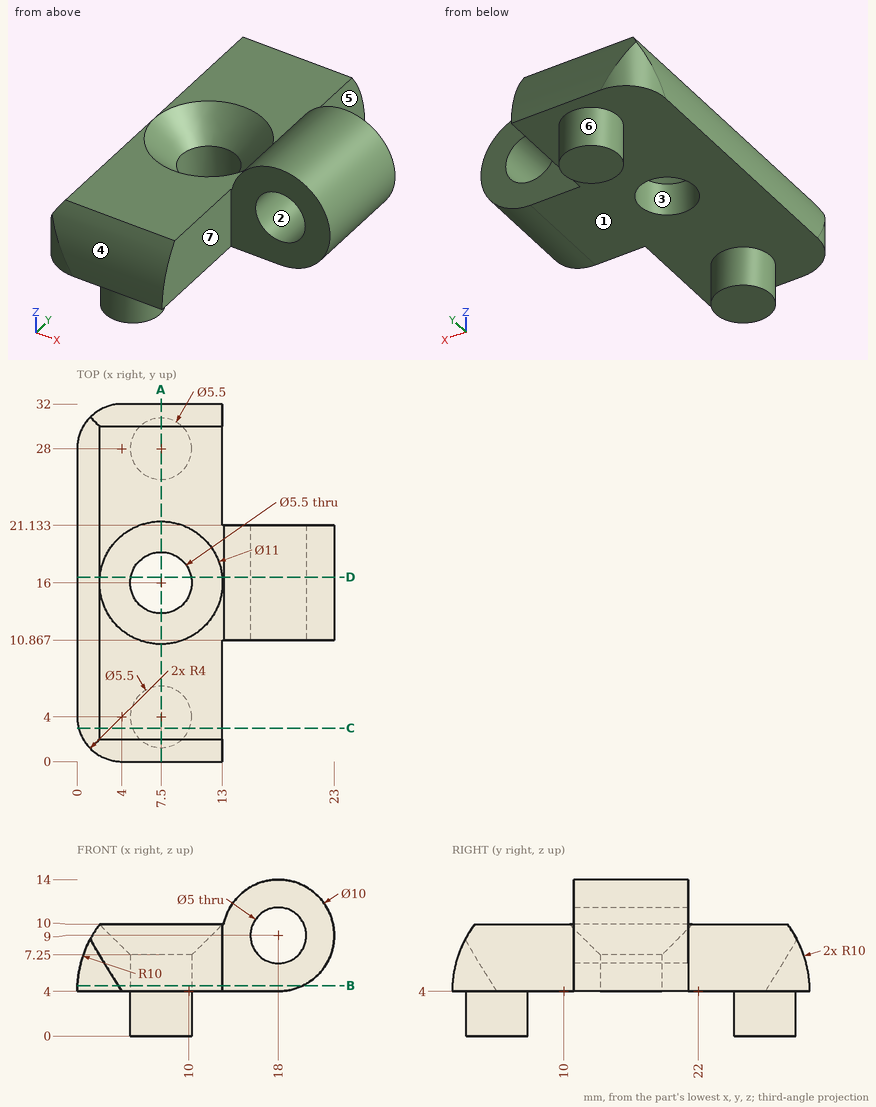
The figure shows three views and two pictorial views of one solid part (mm, origin at its lowest corner). Answer the questions. A direction names the side the tool comes from. Give positions to 0.01 mm unless a question says otherwise; leave off trailing zeros. Loops run counter-clockwise (first coordinate to the right, second up) from the corner with the lowest first, then second, coordinate; pieces in that order, holes last. Notation, with made-up numbers: (81.25, -28.75) - (133.25, -28.75) arc R21 ccw to (133.25, -10.75) - close; hole circle Ø6 at (4, 0.25). An arc over 180 degrees is marked (long way). Use one line per item in the form item = value.
1. Section D-D on y = 16.5 is taken. Count the separate pieces of the cut face and the enclosed holes in it.
Calculated:
separate_pieces = 2
enclosed_holes = 1
2. Section B-B on z = 4.5 is taken. Give the vertices of the cut face in (x, y).
Calculated:
outline = (0.01, 3.68) arc R4 ccw to (3.68, 0.01) - (13, 0.01) - (13, 10.87) - (20.18, 10.87) - (20.18, 21.13) - (13, 21.13) - (13, 31.99) - (3.68, 31.99) arc R4 ccw to (0.01, 28.32) - close; hole circle Ø5.5 at (7.5, 16)
3. Section C-C on y = 3 is taken. Give the vertices of the cut face in (x, z).
Calculated:
outline = (0.13, 4) - (4.94, 4) - (4.94, 0) - (10.06, 0) - (10.06, 4) - (13, 4) - (13, 10) - (2, 10) arc R10 ccw to (0.13, 5.59) - close
4. Section A-A on x = 7.5 is taken. Give the vertices of the cut face in (y, z).
Calculated:
outline = (0, 4) - (1.25, 4) - (1.25, 0) - (6.75, 0) - (6.75, 4) - (13.25, 4) - (13.25, 7.25) - (10.5, 10) - (2, 10) arc R10 ccw to start; (18.75, 4) - (25.25, 4) - (25.25, 0) - (30.75, 0) - (30.75, 4) - (32, 4) arc R10 ccw to (30, 10) - (21.5, 10) - (18.75, 7.25) - close
5. The mould has two halves that part along Z. Classify the marked faces 1, 2 and 3: pulls with the +Z half, pulls with the -Z half, needs draft (parallel to the pull), parting line crosses it, or undercut.
Calculated:
face_1 = pulls with the -Z half
face_2 = undercut
face_3 = needs draft
6. Find the intervals of material crossed by line 1 along Y through (x, z) = (14.25, 10.75); line 2 along X through (y, z) = (16, 6.4); line 3 along Z through (x, y) = (6.25, 10.5), in increasing order. Write a range as [from, to].
Calculated:
line_1 = [10.87, 21.13]
line_2 = [0.29, 4.75], [10.25, 22.27]
line_3 = [4, 10]
7. Given pin 1 Ø3.5 at (x, y) = (5, 10.5) entering from +Z; pin 2 Ø8 at (y, z) = (26.5, 10.5) entering from +X; pin 3 Ø8 at (y, z) = (8, 12) entering from +X; pin 4 Ø10 at (x, y) = (7, 22.5) entering from -Z, each flat-ended and moving along its own axis, determine where each tip first touches the part or whether it passes through.
Calculated:
pin_1 = 10
pin_2 = 13
pin_3 = 23
pin_4 = 0
8. Which of the six approach directions +Z, -Z, +X, -X, +Y, -Y give full straight-line access (tool end or side, diameter ignored) to the marked faces 4, 5, 6 and 7?
Calculated:
face_4 = +Z, +X, -X, -Y
face_5 = +Z, -Z, +X, +Y
face_6 = -Z
face_7 = +Z, -Z, +X, -Y
